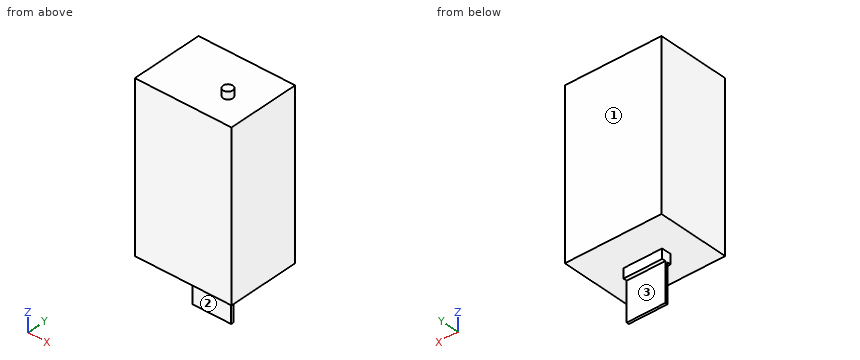
Autodesk Inventor part; units mm, degrees
ref_plane "YZ Plane" through (0, 0, 0) normal (1, 0, 0) x (0, 1, 0)
ref_plane "XZ Plane" through (0, 0, 0) normal (0, 1, 0) x (-1, 0, 0)
ref_plane "XY Plane" through (0, 0, 0) normal (0, 0, 1) x (1, 0, 0)
sketch "Sketch1" plane through (0, 0, 0) normal (0, 1, 0) x (-1, 0, 0)
  line L0 (-10, 34) -> (10, 34)
  line L1 (10, 34) -> (10, 0)
  line L2 (10, 0) -> (-10, 0)
  line L3 (-10, 0) -> (-10, 34)
  line L4 (-4, 0) -> (4, 0)
  line L5 (4, 0) -> (4, -2)
  line L6 (4, -2) -> (-4, -2)
  line L7 (-4, -2) -> (-4, 0)
  line L8 (-4, -2) -> (4, -2)
  line L9 (4, -2) -> (4, -10)
  line L10 (4, -10) -> (-4, -10)
  line L11 (-4, -10) -> (-4, -2)
  dimension "d0" = 20
  dimension "d3" = 2
  dimension "d4" = 8
  dimension "d5" = 44
  dimension "d6" = 34
extrude "Extrusion1" add sketch "Sketch1" along normal blind 15 contours L0 L1 L2 L3
extrude "Extrusion2" add sketch "Sketch1" along normal blind 7 contours L2 L5 L6 L7
extrude "Extrusion3" add sketch "Sketch1" along normal blind 7 contours L6 L9 L10 L11
extrude "Extrusion4" cut sketch "Sketch1" along normal blind 8 contours L2 L5 L6 L7
extrude "Extrusion5" add sketch "Sketch1" along normal blind 8 contours L2 L5 L6 L7
extrude "Extrusion6" cut sketch "Sketch1" along normal blind 6 contours L2 L5 L6 L7
extrude "Extrusion7" add sketch "Sketch1" along normal blind 7.25 contours L6 L9 L10 L11
extrude "Extrusion8" cut sketch "Sketch1" along normal blind 6.75 contours L6 L9 L10 L11
sketch "Sketch2" plane through (-10, 0, 34) normal (0, 0, 1) x (1, 0, 0)
  circle A0 centre (14, 6) radius 1
  point P0 (10, 0)
  dimension "d25" = 2
extrude "Extrusion9" add sketch "Sketch2" along normal blind 1.5
sketch "Sketch3" plane through (10, 0, 34) normal (1, 0, 0) x (0, 0, -1)
  line L0 (0, 0) -> (34, 0)
  line L1 (34, 0) -> (34, 15)
  line L2 (0, 15) -> (34, 15)
  line L3 (0, 0) -> (0, 15)
  dimension "d28" = 15
sketch "Sketch5" plane through (0, 15, 0) normal (0, 1, 0) x (1, 0, 0)
  point P0 (0, 0)
properties part number "VReg"
CAD build for the part. Positions are in the model's coordinates, mm. Face numbers are marked on the shaded views. A direction names the side the tool comes from. Give positions to 0.01 mm unless a question says otherwise; leave off trailing zeros. Order: outer loops, then holes, each group sorted by start corner. A loop starts at its lowest first (then second) coordinate and runs counter-clockwise, first axis right, second up. Notation, with made-up numbers: (-36.75, 36) - (10.25, 36) arc R19 cw to (10.25, 43) - close; hole circle Ø3 at (18, 38). An arc over 180 degrees is marked (long way). Answer in a Markdown table with one row per item.
1. Probe probe 1 along Y at (x, z) = (-0.5, -0.5); probe 2 along Z at (x, y) = (-7.5, 5.5); probe 3 along Y at (x, z) = (1.75, -5). List the from-to ranges inside material, lowest first. Write a range as [from, to].
Data:
| item | result |
|---|---|
| probe 1 | y = [6, 8] |
| probe 2 | z = [0, 34] |
| probe 3 | y = [6.75, 7.25] |
2. Saw through at A-A, the plane z = -2.5. Give the cut face in (x, y), plus the area to 3 significant figures.
Data:
| item | result |
|---|---|
| outline | (-4, 6.75) - (4, 6.75) - (4, 7.25) - (-4, 7.25) - close |
| area | 4.00 mm² |
3. Tool access for the marked faces 1, 2 and 3: list every direction of +Z, -Z, +X, -X, +Y, -Y with a clear straight run to the whole face (end or side of a thin tool).
Data:
| item | result |
|---|---|
| face 1 | +Z, -Z, +X, -X, +Y |
| face 2 | -Z, +X, -X, -Y |
| face 3 | -Z, +X, -X, +Y |
4. Flat gauge pins, fed straight in: pin 1 (0.6 mm diameter, centred on x = 1.5, y = 6.5, fed in from -Z); pin 2 (2.5 mm diameter, centred on x = 1.5, z = -5.5, fed in from -Y); pin 3 (6.5 mm diameter, centred on x = 1.5, z = -4.5, fed in from +Y); pin 4 (5 mm diameter, centred on x = 0, y = 3, fed in from +Z). Where does each tip first touch, or does it go through?
Data:
| item | result |
|---|---|
| pin 1 | stops at z = -10 |
| pin 2 | stops at y = 6.75 |
| pin 3 | stops at y = 8 |
| pin 4 | stops at z = 34 |
5. Saw through at B-B, the plane y = 10. Give the cut face in (x, z), plus the area to 3 significant figures.
Data:
| item | result |
|---|---|
| outline | (-10, 0) - (10, 0) - (10, 34) - (-10, 34) - close |
| area | 680 mm² |
